For this review, take the finished solid that the model builds, in its own axes (mm). A direction names the side the tool comes from. Coordinates: 2 decimals unless noted, no trailing zeros. Loops run counter-clockwise (first coordinate to the right, second up) from the corner with the lowest first, then second, coordinate; pieces in that order, holes last. Notation, with made-up numbers: M 79,-6.5 L 98,-6.5 A13 cw 98,1.5 Z; hole C 78,28.25 d6. An arc over 180 degrees is marked long. Put each result on its own line as item: value.
```python
from build123d import *

# Parameters (mm, degrees)
SKETCH1_R           = 150
BOSS_EXTRUDE1_DEPTH = 150
SKETCH2_R           = 30
CUT_EXTRUDE1_DEPTH  = 50
FILLET1_R           = 20
SKETCH3_R           = 10
CUT_EXTRUDE2_DEPTH  = 5
FILLET4_R           = 50


with BuildPart() as part:
    # Sketch1 → Boss-Extrude1 (new body)
    with BuildSketch(Plane.XY):
        Circle(SKETCH1_R)
    extrude(amount=BOSS_EXTRUDE1_DEPTH)

    # Sketch2 → Cut-Extrude1 (cut)
    with BuildSketch(Plane.XY.offset(150)):
        Circle(SKETCH2_R)
    extrude(amount=-CUT_EXTRUDE1_DEPTH, mode=Mode.SUBTRACT)

    # Fillet1
    fillet1_edges = [part.edges().sort_by_distance(p)[0] for p in [
        (-150, 0, 0),
        (-150, 0, 150),
    ]]
    fillet(fillet1_edges, radius=FILLET1_R)

    # Sketch3 → Cut-Extrude2 (cut)
    with BuildSketch(Plane(origin=(0, 0, 0), x_dir=(-1, 0, 0), z_dir=(0, 0, -1))):
        Circle(SKETCH3_R)
    extrude(amount=-CUT_EXTRUDE2_DEPTH, mode=Mode.SUBTRACT)

    # Fillet4
    # the kernel refuses this fillet: 50 mm, written as the material it takes off along each edge
    with BuildSketch(Plane(origin=(0, 0, 0), x_dir=(-1, 0, 0), z_dir=(0, -1, 0))) as fillet4_piece_1:
        with BuildLine():
            CenterArc((31.794494718, -50), FILLET4_R, 90, 25.841932763)
            Line((10, -5), (9.564110106, -4.1))
            ThreePointArc((9.564110106, -4.1), (9, -2.5), (9, 0))
            Line((9, 0), (10, 1))
            Line((10, 1), (31.794494718, 1))
            Line((31.794494718, 1), (31.794494718, 0))
        make_face()
    revolve(axis=Axis((0, 0, 0), (0, 0, -1)), mode=Mode.SUBTRACT)


solid = part.part
```
(1) Add section C-C (z = 10). Write out the cut boundary in (x, y).
Determined:
outline: C 0,0 d294.64
(2) Add section B-B (z = 90.5). Write out the cut boundary in (x, y).
Determined:
outline: C 0,0 d300
(3) Draft analysis for pull direction Y (two halves, no side actions). For faces 1 (the cylindrical face through (-29.97, 1.32, 125.35)), 2 (the cylindrical face through (-19.527, 148.724, 74.23)), 3 (the flat face through (-2, 31, 150)), state which applies: +Y half, -Y half, draft (parallel to the pull), parting line (faces both ways), or undercut.
Determined:
face 1: undercut
face 2: parting line
face 3: draft
(4) Wall thickness on line 1 along Y through (x, z) = (0, 130); line 2 along X through (y, z) = (96, 46); line 3 along Y through (x, z) = (125, 136): over which ranges is each line inside the solid? List them lowest first. Write a range as [from, to].
Determined:
line 1: y = [-150, -30], [30, 150]
line 2: x = [-115.26, 115.26]
line 3: y = [-81.24, 81.24]
(5) Tool access review of faces 4 (the flat face through (27, -27, 0)), 5 (the flat face through (0, 0, 5)), 6 (the flat face through (0, 0, 100)): name each direction out of +Z, -Z, +X, -X, +Y, -Y from which nothing blocks a thin tool from reaching the whole face with its end or side.
Determined:
face 4: -Z, +X, -X, +Y, -Y
face 5: -Z
face 6: +Z
(6) For pin 1 (2 mm diameter, centred on y = 72.5, z = 102.5, fed in from -X); pin 2 (1.5 mm diameter, centred on x = 114.5, y = -79.5, fed in from +Z); pin 3 (3 mm diameter, centred on x = -74.5, z = 111, fed in from -Y), all flat-tipped, find the tip position at first contact; note any pin that passes through.
Determined:
pin 1: stops at x = -131.86
pin 2: stops at z = 148.04
pin 3: stops at y = -131.04
(7) Add section A-A (z = 123.5). Write out the cut boundary in (x, y), plus the area to 3 significant figures.
Determined:
outline: C 0,0 d300; hole C 0,0 d60
area: 67,900 mm^2
